from build123d import *

# Parameters (mm, degrees)
SKETCH_1_W          = 45
SKETCH_1_H          = 45
EXTRUDE_1_DEPTH     = 12
SKETCH_2_W          = 6
SKETCH_2_H          = 38
CUT_EXTRUDE_1_DEPTH = 52.722818949
SKETCH_3_R          = 3
SKETCH_3_R_2        = 1.5
CUT_EXTRUDE_2_DEPTH = 35.007352146
SKETCH_4_R          = 1.5
CUT_EXTRUDE_3_DEPTH = 35.007352146
SKETCH_6_W          = 7
SKETCH_6_H          = 12
CUT_EXTRUDE_4_DEPTH = 7
SKETCH_7_W          = 30
SKETCH_7_H          = 20
SKETCH_7_W_2        = 8
EXTRUDE_2_DEPTH     = 9.2
SKETCH_9_W          = 30
SKETCH_9_H          = 20
EXTRUDE_4_DEPTH     = 3


with BuildPart() as part:
    # Sketch 1 → Extrude 1 (new body)
    with BuildSketch(Plane.XY):
        Rectangle(SKETCH_1_W, SKETCH_1_H)
    extrude(amount=EXTRUDE_1_DEPTH)

    # Sketch 2 → Cut-Extrude 1 (cut, through all)
    with BuildSketch(Plane.ZY.offset(22.5)):
        with Locations((6, 3.5)):
            Rectangle(SKETCH_2_W, SKETCH_2_H)
    extrude(amount=-CUT_EXTRUDE_1_DEPTH, mode=Mode.SUBTRACT)

    # Sketch 3 → Cut-Extrude 2 (cut, through all)
    with BuildSketch(Plane.XY.offset(12)):
        with Locations((-12, 16.5)):
            Circle(SKETCH_3_R)
        with Locations((12, 16.5)):
            Circle(SKETCH_3_R_2)
    extrude(amount=-CUT_EXTRUDE_2_DEPTH, mode=Mode.SUBTRACT)

    # Sketch 4 → Cut-Extrude 3 (cut, through all)
    with BuildSketch(Plane.XY.offset(12)):
        with Locations((-12, -3.5)):
            Circle(SKETCH_4_R)
        with Locations((12, -3.5)):
            Circle(SKETCH_4_R)
    extrude(amount=-CUT_EXTRUDE_3_DEPTH, mode=Mode.SUBTRACT)

    # Sketch 6 → Cut-Extrude 4 (cut)
    with BuildSketch(Plane.XZ.offset(22.5)):
        with Locations((-19, 6)):
            Rectangle(SKETCH_6_W, SKETCH_6_H)
        with Locations((19, 6)):
            Rectangle(SKETCH_6_W, SKETCH_6_H)
    extrude(amount=-CUT_EXTRUDE_4_DEPTH, mode=Mode.SUBTRACT)

    # Sketch 7 → Extrude 2 (add)
    with BuildSketch(Plane(origin=(0, 0, 0), x_dir=(-1, 0, 0), z_dir=(0, 0, -1))):
        with Locations((37.5, 12.5)):
            Rectangle(SKETCH_7_W, SKETCH_7_H)
        with Locations((-1.8, 12.5)):
            Rectangle(SKETCH_7_W_2, SKETCH_7_H)
    extrude(amount=EXTRUDE_2_DEPTH)


with BuildPart() as extrude_2_piece_1:
    # of the separate pieces the step leaves, piece 1, a body of its own (extrude_2_pieces)
    add(part.part.solids().sort_by_distance((15.5, -22.5, 0))[0])



with BuildPart() as extrude_2_piece_2:
    # of the separate pieces the step leaves, piece 2, a body of its own (extrude_2_pieces)
    add(part.part.solids().sort_by_distance((-22.5, 2.5, -9.2))[0])


with BuildPart() as extrude_2_piece_1_1:
    add(extrude_2_piece_1.part)

    add(extrude_2_piece_2.part)  # Extrude 4 merges Extrude 2 piece 2
    # Sketch 9 → Extrude 4 (add)
    with BuildSketch(Plane.XY):
        with Locations((-37.5, 12.5)):
            Rectangle(SKETCH_9_W, SKETCH_9_H)
    extrude(amount=EXTRUDE_4_DEPTH)


solid = extrude_2_piece_1_1.part
Geometry check sheet. Reference: the model listing, model coordinates, mm. A direction names the side the tool comes from. Coordinates: 2 decimals unless noted, no trailing zeros. Order: outer loops, then holes, each group sorted by start corner. A loop starts at its lowest first (then second) coordinate and runs counter-clockwise, first axis right, second up. Notation, with made-up numbers: (4.25, 23) -> (14.25, 23) arc R15 cw to (14.25, 36) -> close; hole circle Ø2 at (5, 81.5). An arc over 180 degrees is marked (long way). Use a Markdown table: item, result. Add a question column.
1. Cross-section at B-B (y = -13). Enter the section's corners in (x, z).
2. Cross-section at C-C (x = 12). Enter the section's corners in (y, z).
3. Cross-section at A-A (y = -3.5). Enter the section's corners in (x, z), and give its area (3 significant figures).
4. Go/stop test with flat-tipped pins: pin 1 Ø7.5 at (y, z) = (-19.5, 7) entering from -X; pin 2 Ø1.5 at (y, z) = (-5, 2) entering from -X; pin 3 Ø2.5 at (x, z) = (-20, 1) entering from -Y; pin 4 Ø1.5 at (x, z) = (-24, 9) entering from -Y. Record where each tip stops, or that it passes through.
5. Material ranges on L1, parallel to Y at x = -12, z = 9.95; L2, parallel to Y at x = 12, z = 10.6; L3, parallel to Z at x = 4, y = 4.5, recorded low to high.
6. Mould release check, pull along Z, two halves, no side actions. Record for faces 4 (the face through (-52.5, 12, -3)), 5 (the face through (-7, 8, 3)), 6 (the face through (2, 13, -9.2)): pulls with the +Z half, pulls with the -Z half, needs draft (parallel to the pull), parting line crosses it, or undercut.
7. Cross-section at D-D (z = 2). Enter the section's corners in (x, y).
8. Set-up check for faces 1 (the face through (15.5, -19, 6)), 2 (the face through (0, -15.5, 6)), 3 (the face through (-22.5, -7, 1)): record each of +Z, -Z, +X, -X, +Y, -Y from which the full face is reachable in a straight line by a thin tool's end or side.
Filled sheet:
| question | item | result |
|---|---|---|
| 1 | outline | (-22.5, 0) -> (22.5, 0) -> (22.5, 3) -> (-22.5, 3) -> close; (-22.5, 9) -> (22.5, 9) -> (22.5, 12) -> (-22.5, 12) -> close |
| 2 | outline | (-22.5, 0) -> (-5, 0) -> (-5, 3) -> (-15.5, 3) -> (-15.5, 9) -> (-5, 9) -> (-5, 12) -> (-22.5, 12) -> close; (-2, 0) -> (15, 0) -> (15, 3) -> (-2, 3) -> close; (-2, 9) -> (15, 9) -> (15, 12) -> (-2, 12) -> close; (18, 0) -> (22.5, 0) -> (22.5, 3) -> (18, 3) -> close; (18, 9) -> (22.5, 9) -> (22.5, 12) -> (18, 12) -> close |
| 3 | outline | (-22.5, 0) -> (-13.5, 0) -> (-13.5, 3) -> (-22.5, 3) -> close; (-22.5, 9) -> (-13.5, 9) -> (-13.5, 12) -> (-22.5, 12) -> close; (-10.5, 0) -> (10.5, 0) -> (10.5, 3) -> (-10.5, 3) -> close; (-10.5, 9) -> (10.5, 9) -> (10.5, 12) -> (-10.5, 12) -> close; (13.5, 0) -> (22.5, 0) -> (22.5, 3) -> (13.5, 3) -> close; (13.5, 9) -> (22.5, 9) -> (22.5, 12) -> (13.5, 12) -> close |
| 3 | area | 234 mm2 |
| 4 | pin 1 | x = -15.5 |
| 4 | pin 2 | x = -22.5 |
| 4 | pin 3 | y = -15.5 |
| 4 | pin 4 | through |
| 5 | L1 | -22.5 to -5, -2 to 13.5, 19.5 to 22.5 |
| 5 | L2 | -22.5 to -5, -2 to 15, 18 to 22.5 |
| 5 | L3 | -9.2 to 3, 9 to 12 |
| 6 | face 4 | needs draft |
| 6 | face 5 | undercut |
| 6 | face 6 | pulls with the -Z half |
| 7 | outline | (-52.5, 2.5) -> (-22.5, 2.5) -> (-22.5, -15.5) -> (-15.5, -15.5) -> (-15.5, -22.5) -> (15.5, -22.5) -> (15.5, -15.5) -> (22.5, -15.5) -> (22.5, 22.5) -> (-52.5, 22.5) -> close; hole circle Ø6 at (-12, 16.5); hole circle Ø3 at (-12, -3.5); hole circle Ø3 at (12, -3.5); hole circle Ø3 at (12, 16.5) |
| 8 | face 1 | +Z, -Z, +X, -Y |
| 8 | face 2 | +X, -X, +Y |
| 8 | face 3 | +Z, -Z, -X, -Y |
